Check sheet for the modelled part. Datum: model origin and axes. Units: mm. A direction names the side the tool comes from. Round coordinates to 2 decimals unless told otherwise and drop trailing zeros. Order: outer loops, then holes, each group sorted by start corner. A loop starts at its lowest first (then second) coordinate and runs counter-clockwise, first axis right, second up.
Q1. Set-up check for faces 5 (the flat face through (-12.5, -8, 11)), 6 (the flat face through (-2, 12.5, 2)), 7 (the flat face through (-8, -7.5, 15)): record each of +Z, -Z, +X, -X, +Y, -Y from which the full face is reachable in a straight line by a thin tool's end or side.
Q2. Scan lines: probe 1 along Z at (x, y) = (-1.75, -7); probe 2 along X at (y, z) = (10, 13.5); probe 3 along Y at (x, z) = (-8.5, 14.5). Record each from-to range of solid material in increasing order.
Q3. Cross-section at D-D on y = 15. Record the cut outline in (x, z), then the cut area to 3 significant figures.
Q4. Depth check by flat-ended pin: P1, Ø10, axis at x = -8, y = 14, coming from the -Z side; P2, Ø2, axis at x = 4.5, z = 5.5, coming from the -Y side; P3, Ø5.5, axis at x = -5.5, z = 28.5, coming from the +Y side; P4, Ø1.5, axis at y = 17.5, z = 19.5, coming from the -X side. Enter the tip coordinate at first touch or a pass-through.
Q5. Cross-section at C-C on y = 8. Record the cut outline in (x, z).
Q6. Cross-section at A-A on x = -8.75. Record the cut outline in (y, z).
Q7. Mould release check, pull along Z, two halves, no side actions. Record for faces 1 (the cylindrical face through (4.65, -4.49, 14.86)), 2 (the flat face through (12.5, 15, 15)), 3 (the flat face through (0, 3, 30)), 4 (the flat face through (0, 3, 0)): +Z half, -Z half, draft (parallel to the pull), parting line (faces both ways), or undercut.
Q8. Cross-section at B-B on z = 3. Record the cut outline in (x, y).
Autodesk Inventor part; units mm, degrees
ref_plane "YZ Plane" through (0, 0, 0) normal (1, 0, 0) x (0, 1, 0)
ref_plane "XZ Plane" through (0, 0, 0) normal (0, 1, 0) x (-1, 0, 0)
ref_plane "XY Plane" through (0, 0, 0) normal (0, 0, 1) x (1, 0, 0)
sketch "Esboço1" plane through (0, 0, 0) normal (0, 0, 1) x (1, 0, 0)
  line L0 (-12.5, -12.5) -> (-2.5, -12.5)
  line L1 (12.5, 2.5) -> (12.5, 12.5)
  line L2 (12.5, 12.5) -> (-12.5, 12.5)
  line L3 (-12.5, 12.5) -> (-12.5, -12.5)
  line L4 (-12.5, -12.5) -> (12.5, 12.5) construction
  line L5 (12.5, -12.5) -> (-12.5, 12.5) construction
  line L6 (12.5, 12.5) -> (7.5, 12.5)
  line L7 (7.5, 12.5) -> (7.5, 27.5)
  line L8 (7.5, 27.5) -> (12.5, 27.5)
  line L9 (12.5, 27.5) -> (12.5, 12.5)
  arc A0 (-2.5, -12.5) -> (12.5, 2.5) centre (-2.5, 2.5) ccw
  point P0 (0, 0)
  dimension "d0" = 25
  dimension "d1" = 25
  dimension "d2" = 5
  dimension "d3" = 15
  dimension "d4" = 15
extrude "Extrusão1" add sketch "Esboço1" along normal blind 30
shell "Casca1" thickness 5 removed faces 2 at (0.8333, 12.5, 10) at (-12.5, 4.1667, 20)
properties part number "Servo mount"
Results found:
1. face 5: +Z, -Z, -X, +Y, -Y
1. face 6: +Z, -Z, -X, +Y
1. face 7: -X, +Y
2. probe 1: z = 0 to 5, 25 to 30
2. probe 2: x = 7.5 to 12.5
2. probe 3: y = -12.5 to -7.5
3. outline: (7.5, 0) - (12.5, 0) - (12.5, 30) - (7.5, 30) - close
3. area: 150 mm2
4. P1: stops at z = 0
4. P2: stops at y = -11.25
4. P3: stops at y = 12.5
4. P4: stops at x = 7.5
5. outline: (-12.5, 0) - (12.5, 0) - (12.5, 30) - (-12.5, 30) - (-12.5, 25) - (7.5, 25) - (7.5, 5) - (-12.5, 5) - close
6. outline: (-12.5, 0) - (12.5, 0) - (12.5, 5) - (-7.5, 5) - (-7.5, 25) - (12.5, 25) - (12.5, 30) - (-12.5, 30) - close
7. face 1: undercut
7. face 2: draft
7. face 3: +Z half
7. face 4: -Z half
8. outline: (-12.5, -12.5) - (-2.5, -12.5) arc R15 ccw to (12.5, 2.5) - (12.5, 27.5) - (7.5, 27.5) - (7.5, 12.5) - (-12.5, 12.5) - close
